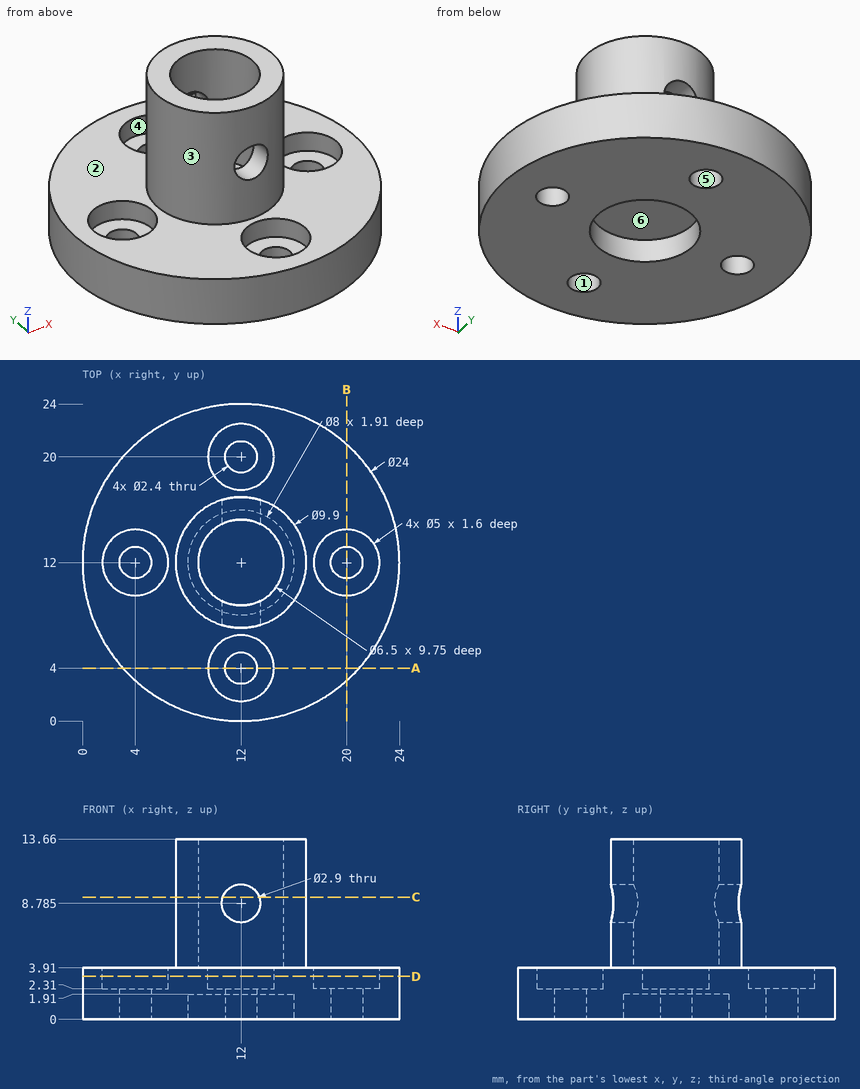
Part print with two shaded views. Sizes in mm from the minimum x, y, z corner. A direction names the side the tool comes from. Coordinates: 2 decimals unless noted, no trailing zeros. Order: outer loops, then holes, each group sorted by start corner. A loop starts at its lowest first (then second) coordinate and runs counter-clockwise, first axis right, second up.
(1) Pin check, flat tips, straight feed: pin 1 Ø2 at (x, y) = (21, 11.5) entering from +Z; pin 2 Ø4.5 at (x, z) = (12, 8.785) entering from -Y; pin 3 Ø1.5 at (y, z) = (11.5, 9.5) entering from +X; pin 4 Ø2 at (x, y) = (12, 20) entering from -Z. Stop position of each tip, or through.
Solution:
pin 1: stops at z = 2.31
pin 2: stops at y = 7.05
pin 3: stops at x = 16.95
pin 4: passes through
(2) Saw through at D-D, the plane z = 3.25. Write the cut outline in (x, y).
Solution:
outline: circle Ø24 at (12, 12); hole circle Ø5 at (4, 12); hole circle Ø5 at (12, 4); hole circle Ø5 at (12, 20); hole circle Ø5 at (20, 12)
(3) Drill centre lines: L1, parallel to Y at x = 12, z = 3.45; L2, parallel to Y at x = 12, z = 1; L3, parallel to Z at x = 13.75, y = 16.75. Where is each one in solid material? Low to high.
Solution:
L1: y = 0 to 1.5, 6.5 to 17.5, 22.5 to 24
L2: y = 0 to 2.8, 5.2 to 8, 16 to 18.8, 21.2 to 24
L3: z = 0 to 3.91
(4) Saw through at A-A, the plane y = 4. Write the cut outline in (x, z), and give its area (3 significant figures).
Solution:
outline: (3.06, 0) - (10.8, 0) - (10.8, 2.31) - (9.5, 2.31) - (9.5, 3.91) - (3.06, 3.91) - close; (13.2, 0) - (20.94, 0) - (20.94, 3.91) - (14.5, 3.91) - (14.5, 2.31) - (13.2, 2.31) - close
area: 56.4 mm2
(5) Mould opens along X. For the marked faces 1, 2 and 3 say: released by +X, released by -X, zero draft, split by the parting line, or undercut.
Solution:
face 1: undercut
face 2: zero draft
face 3: split by the parting line
(6) Which spindle directions (+Z, -Z, +X, -X, +Y, -Y) get a long thin tool onto all of the face, cutting with end or side? Do the marked faces 4, 5 and 6. Say none if no direction does.
Solution:
face 4: +Z
face 5: +Z, -Z
face 6: -Z
(7) Saw through at C-C, the plane z = 9.25. Write the cut outline in (x, y), and give its area (3 significant figures).
Solution:
outline: (10.63, 7.24) - (10.63, 9.05) arc R3.25 cw to (10.63, 14.95) - (10.63, 16.76) arc R4.95 ccw to start; (13.37, 7.24) arc R4.95 ccw to (13.37, 16.76) - (13.37, 14.95) arc R3.25 cw to (13.37, 9.05) - close
area: 34.3 mm2
